Check sheet for the modelled part. Datum: model origin and axes. Units: mm. A direction names the side the tool comes from. Round coordinates to 2 decimals unless told otherwise and drop trailing zeros. Write each loop counter-clockwise with the first axis right and the second up, starting at its lowest first coordinate (ties: lowest second). Pieces come first, ordered by that corner, then holes. Notation, with made-up numbers: (84.5, 4.25) - (136.5, 4.25) arc R11 ccw to (136.5, 23.25) - close; hole circle Ø5 at (4.25, 28.5). An arc over 180 degrees is marked (long way). Answer as a JSON object with one key per item and string values. Group by question number.
Item 1: Release check for a two-part mould opening along Z. For faces 5 (the flat face through (5.5, 3, 15)), 6 (the flat face through (7, 7, -35)), 7 (the flat face through (1.4, 5.6, -39.8)) record: pulls with the +Z half, pulls with the -Z half, needs draft (parallel to the pull), parting line crosses it, or undercut.
Item 2: Gauge pin test, flat ends, axial feed: P1, Ø1.5, axis at x = 7, y = 8.5, coming from the +Z side; P2, Ø5.5, axis at y = 5.5, z = -29, coming from the +X side; P3, Ø5.5, axis at x = 9, y = 9.5, coming from the -Z side. Record the tip position at first contact, or that the pin passes through.
Item 3: Sectioned sample at D-D on z = -30. Record the boundary of the cut face in (x, y).
Item 4: Sectioned sample at C-C on y = 2. Record the boundary of the cut face in (x, z).
Item 5: Sectioned sample at B-B on z = -19. Record the boundary of the cut face in (x, y), plus the area to 3 significant figures.
Item 6: Sectioned sample at A-A on x = 9.75. Record the boundary of the cut face in (y, z), plus the area to 3 significant figures.
Item 7: Thickness scan on line 1 (Z direction, x = 14.25, y = 7.5); line 2 (Z direction, x = 4.25, y = 4.25); line 3 (Y direction, x = 8.25, z = 13.5). Record the ranges inside material, lowest first.
Item 8: Set-up check for faces 1 (the flat face through (14.7, 5.6, -10)), 2 (the flat face through (8, 9, -40)), 3 (the cylindrical face through (-4.73, 7.51, -30.14)), 4 (the flat face through (8, 6, 0)): record each of +Z, -Z, +X, -X, +Y, -Y from which the full face is reachable in a straight line by a thin tool's end or side.
```python
from build123d import *

# Parameters (mm, degrees)
SKETCH1_W             = 10.6165
SKETCH1_H             = 20
SKETCH1_W_2           = 10.732
SKETCH1_H_2           = 10
BOSS_EXTRUDE1_DEPTH   = 6
SKETCH2_W             = 10.6165
SKETCH2_H             = 5
BOSS_EXTRUDE2_DEPTH   = 5
CHAMFER1_SIZE         = 2
BOSS_EXTRUDE3_START   = -10
SKETCH3_R             = 4.95
BOSS_EXTRUDE3_DEPTH   = 20
BOSS_EXTRUDE4_START   = 10
SKETCH3_3_R           = 4.95
BOSS_EXTRUDE4_DEPTH   = 10
BOSS_EXTRUDE5_START   = -20
SKETCH3_4_R           = 4.95
BOSS_EXTRUDE5_DEPTH   = 10
BOSS_EXTRUDE6_START   = -40
SKETCH3_5_R           = 4.95
BOSS_EXTRUDE6_DEPTH   = 20
BOSS_EXTRUDE7_START   = -50
SKETCH3_6_R           = 4.95
BOSS_EXTRUDE7_DEPTH   = 10
F_1_0MM_DOWEL_HOLE1_D = 2.5
CUT_EXTRUDE1_START    = -0.2
CUT_EXTRUDE1_DEPTH    = 0.2
CUT_EXTRUDE2_START    = -30.2
CUT_EXTRUDE2_DEPTH    = 10.4
CUT_EXTRUDE3_START    = -50
CUT_EXTRUDE3_DEPTH    = 0.2


with BuildPart() as part:
    # Sketch1 → Boss-Extrude1 (new body)
    with BuildSketch(Plane(origin=(0, 0, 0), x_dir=(1, 0, 0), z_dir=(0, 1, 0))):
        Polygon((16.2325, -10), (10.6165, -10), (5.5005, -10), (5.5005, -20), (16.2325, -20), align=None)
        Polygon((10.6165, 0), (0, 0), (0, -10), (5.5005, -10), (10.6165, -10), align=None)
        Polygon((0, 10), (0, 0), (10.6165, 0), (10.6165, 10), (5.5005, 10), align=None)
        Polygon((5.5005, 10), (10.6165, 10), (16.2325, 10), (16.2325, 20), (10.6165, 20), (5.5005, 20), align=None)
        with Locations((5.30825, 30)):
            Rectangle(SKETCH1_W, SKETCH1_H)
        with Locations((10.8665, 45)):
            Rectangle(SKETCH1_W_2, SKETCH1_H_2)
    extrude(amount=BOSS_EXTRUDE1_DEPTH)

    # Sketch2 → Boss-Extrude2 (add)
    with BuildSketch(Plane(origin=(0, 6, 0), x_dir=(1, 0, 0), z_dir=(0, 1, 0))):
        with Locations((5.30825, 7.5)):
            Rectangle(SKETCH2_W, SKETCH2_H)
        with Locations((5.30825, -7.5)):
            Rectangle(SKETCH2_W, SKETCH2_H)
        with Locations((5.30825, 37.5)):
            Rectangle(SKETCH2_W, SKETCH2_H)
        with Locations((5.30825, 22.5)):
            Rectangle(SKETCH2_W, SKETCH2_H)
    extrude(amount=BOSS_EXTRUDE2_DEPTH)

    # Chamfer1
    chamfer1_edges = [part.edges().sort_by_distance(p)[0] for p in [
        (5.30825, 11, -35),
        (5.30825, 11, -25),
        (5.30825, 11, -5),
        (5.30825, 11, 5),
    ]]
    chamfer(chamfer1_edges, length=CHAMFER1_SIZE)

    # Sketch3 → Boss-Extrude3 (add)
    with BuildSketch(Plane.XY.offset(BOSS_EXTRUDE3_START)):
        with Locations((0, 6.05)):
            Circle(SKETCH3_R)
    extrude(amount=BOSS_EXTRUDE3_DEPTH)

    # Sketch3<3> → Boss-Extrude4 (add)
    with BuildSketch(Plane.XY.offset(BOSS_EXTRUDE4_START)):
        with Locations((16.2325, 6.05)):
            Circle(SKETCH3_3_R)
    extrude(amount=BOSS_EXTRUDE4_DEPTH)

    # Sketch3<4> → Boss-Extrude5 (add)
    with BuildSketch(Plane.XY.offset(BOSS_EXTRUDE5_START)):
        with Locations((16.2325, 6.05)):
            Circle(SKETCH3_4_R)
    extrude(amount=BOSS_EXTRUDE5_DEPTH)

    # Sketch3<5> → Boss-Extrude6 (add)
    with BuildSketch(Plane.XY.offset(BOSS_EXTRUDE6_START)):
        with Locations((0, 6.05)):
            Circle(SKETCH3_5_R)
    extrude(amount=BOSS_EXTRUDE6_DEPTH)

    # Sketch3<6> → Boss-Extrude7 (add)
    with BuildSketch(Plane.XY.offset(BOSS_EXTRUDE7_START)):
        with Locations((16.2325, 6.05)):
            Circle(SKETCH3_6_R)
    extrude(amount=BOSS_EXTRUDE7_DEPTH)

    # Ø1.0mm Dowel Hole1 (through all)
    with Locations(Plane.XY.offset(20)):
        with Locations((0, 6.05), (16.2325, 6.05)):
            Hole(F_1_0MM_DOWEL_HOLE1_D / 2)

    # Sketch9 → Cut-Extrude1 (cut)
    with BuildSketch(Plane.XY.offset(10).offset(CUT_EXTRUDE1_START)):
        with BuildLine():
            Line((5.5005, 6), (5.5005, 11))
            Line((5.5005, 11), (0, 11))
            ThreePointArc((0, 11), (-4.95, 6.05), (0, 1.1))
            Line((0, 1.1), (0, 0))
            Line((0, 0), (5.5005, 0))
            Line((5.5005, 0), (5.5005, 6))
        make_face()
    extrude(amount=CUT_EXTRUDE1_DEPTH, mode=Mode.SUBTRACT)

    # Sketch9<2> → Cut-Extrude2 (cut)
    with BuildSketch(Plane.XY.offset(10).offset(CUT_EXTRUDE2_START)):
        with BuildLine():
            Line((5.5005, 0), (5.5005, 6))
            Line((5.5005, 6), (5.5005, 11))
            Line((5.5005, 11), (0, 11))
            ThreePointArc((0, 11), (-4.95, 6.05), (0, 1.1))
            Line((0, 1.1), (0, 0))
            Line((0, 0), (5.5005, 0))
        make_face()
    extrude(amount=CUT_EXTRUDE2_DEPTH, mode=Mode.SUBTRACT)

    # Sketch9<4> → Cut-Extrude3 (cut)
    with BuildSketch(Plane.XY.offset(10).offset(CUT_EXTRUDE3_START)):
        with BuildLine():
            Line((5.5005, 0), (5.5005, 6))
            Line((5.5005, 6), (5.5005, 11))
            Line((5.5005, 11), (0, 11))
            ThreePointArc((0, 11), (-4.95, 6.05), (0, 1.1))
            Line((0, 1.1), (0, 0))
            Line((0, 0), (5.5005, 0))
        make_face()
    extrude(amount=CUT_EXTRUDE3_DEPTH, mode=Mode.SUBTRACT)


solid = part.part
```
Completed:
{
 "1": {"face 5": "needs draft", "face 6": "undercut", "face 7": "pulls with the -Z half"},
 "2": {"P1": "z = 10", "P2": "x = 10.62", "P3": "z = -40"},
 "3": {"outline": "(0, 0) - (10.62, 0) - (10.62, 6) - (4.95, 6) arc R4.95 ccw (long way) to (0, 1.1) - close; hole circle Ø2.5 at (0, 6.05)"},
 "4": {"outline": "(-2.85, -39.8) - (5.5, -39.8) - (5.5, -50) - (19.08, -50) - (19.08, -40) - (10.62, -40) - (10.62, -20) - (19.08, -20) - (19.08, -10) - (10.62, -10) - (10.62, 10) - (19.08, 10) - (19.08, 20) - (5.5, 20) - (5.5, 9.8) - (-2.85, 9.8) - (-2.85, -9.8) - (5.5, -9.8) - (5.5, -20.2) - (-2.85, -20.2) - close"},
 "5": {"outline": "(5.5, 0) - (16.23, 0) - (16.23, 1.1) arc R4.95 ccw (long way) to (11.28, 6) - (5.5, 6) - close; hole circle Ø2.5 at (16.23, 6.05)", "area": "117 mm²"},
 "6": {"outline": "(0, -50) - (6, -50) - (6, -40) - (11, -40) - (11, -37) - (9, -35) - (6, -35) - (6, -25) - (9, -25) - (11, -23) - (11, -20) - (6, -20) - (6, -10) - (11, -10) - (11, -7) - (9, -5) - (6, -5) - (6, 5) - (9, 5) - (11, 7) - (11, 10) - (6, 10) - (6, 20) - (0, 20) - close", "area": "512 mm²"},
 "7": {"line 1": "-50 to -40, -20 to -10, 10 to 20", "line 2": "-39.8 to -20.2, -9.8 to 9.8", "line 3": "0 to 6"},
 "8": {"face 1": "+X, +Y, -Y", "face 2": "-Z, -X, +Y", "face 3": "none", "face 4": "+X, +Y"}
}
